```python
from build123d import *

# Parameters (mm, degrees)
SKETCH1_W           = 5.54
SKETCH1_H           = 6.3
BOSS_EXTRUDE1_DEPTH = 8.8
SKETCH2_W           = 0.8
SKETCH2_H           = 0.5
BOSS_EXTRUDE2_DEPTH = 3.2
CUT_EXTRUDE1_REACH  = 7.54
SKETCH4_W           = 2
SKETCH4_H           = 4
CUT_EXTRUDE2_DEPTH  = 3.15
CUT_EXTRUDE2_TAPER  = 10


with BuildPart() as part:
    # Sketch1 → Boss-Extrude1 (new body)
    with BuildSketch(Plane(origin=(0, 0, 0), x_dir=(1, 0, 0), z_dir=(0, 1, 0))):
        Rectangle(SKETCH1_W, SKETCH1_H)
    extrude(amount=BOSS_EXTRUDE1_DEPTH)

    # Sketch2 → Boss-Extrude2 (add)
    with BuildSketch(Plane(origin=(0, 0, 0), x_dir=(1, 0, 0), z_dir=(0, 1, 0))):
        with Locations((1.27, 0.2)):
            Rectangle(SKETCH2_W, SKETCH2_H)
        with Locations((-1.27, 0.2)):
            Rectangle(SKETCH2_W, SKETCH2_H)
    extrude(amount=-BOSS_EXTRUDE2_DEPTH)

    # Sketch3 → Cut-Extrude1 (cut, up to next)
    with BuildSketch(Plane(origin=(2.77, 0, 0), x_dir=(0, 0, -1), z_dir=(1, 0, 0)), mode=Mode.PRIVATE) as cut_extrude1_sk1:
        with BuildLine():
            ThreePointArc((-3.15, 4.7), (-2.974264069, 5.124264069), (-2.55, 5.3))
            Line((-2.55, 5.3), (-2.337822174, 5.3))
            Line((-2.337822174, 5.3), (-1.4, 8.8))
            Line((-1.4, 8.8), (-3.15, 8.8))
            Line((-3.15, 8.8), (-3.15, 4.7))
        make_face()
    cut_extrude1_tool1 = extrude(cut_extrude1_sk1.sketch, amount=-CUT_EXTRUDE1_REACH, mode=Mode.PRIVATE) & part.part
    add(cut_extrude1_tool1.solids().sort_by_distance((2.77, 7.227986, 2.489914))[0], mode=Mode.SUBTRACT)
    # Sketch3 → Cut-Extrude1 (cut, up to next)
    with BuildSketch(Plane(origin=(2.77, 0, 0), x_dir=(0, 0, -1), z_dir=(1, 0, 0)), mode=Mode.PRIVATE) as cut_extrude1_sk2:
        Polygon((3.15, 8.8), (1.4, 8.8), (3.15, 2.268911087), align=None)
    cut_extrude1_tool2 = extrude(cut_extrude1_sk2.sketch, amount=-CUT_EXTRUDE1_REACH, mode=Mode.PRIVATE) & part.part
    add(cut_extrude1_tool2.solids().sort_by_distance((2.77, 6.62297, -2.566667))[0], mode=Mode.SUBTRACT)

    # Sketch4 → Cut-Extrude2 (cut)
    with BuildSketch(Plane.XY.offset(3.15)):
        with Locations((-1.27, 2.268911087)):
            Rectangle(SKETCH4_W, SKETCH4_H)
        with Locations((1.27, 2.268911087)):
            Rectangle(SKETCH4_W, SKETCH4_H)
    extrude(amount=-CUT_EXTRUDE2_DEPTH, taper=CUT_EXTRUDE2_TAPER, mode=Mode.SUBTRACT)


solid = part.part
```
The listing builds one solid part. Answer for the finished solid, in the listing's coordinates (mm). A direction names the side the tool comes from. Coordinates: 2 decimals unless noted, no trailing zeros. Write each loop counter-clockwise with the first axis right and the second up, starting at its lowest first coordinate (ties: lowest second). Pieces come first, ordered by that corner, then holes. Notation, with made-up numbers: (0.5, 21) - (55.5, 21) arc R28 ccw to (55.5, 59) - close; hole circle Ø6 at (-9.75, -14). An arc over 180 degrees is marked (long way). One line per item, written item: value.
1) Find section A-A (y = -0.25). Give the vertices of the cut face in (x, z), and give its area (3 significant figures).
Geometry check:
outline: (-1.67, -0.45) - (-0.87, -0.45) - (-0.87, 0.05) - (-1.67, 0.05) - close; (0.87, -0.45) - (1.67, -0.45) - (1.67, 0.05) - (0.87, 0.05) - close
area: 0.800 mm2
2) Find section B-B (z = -0.25). Give the vertices of the cut face in (x, y), and give its area (3 significant figures).
Geometry check:
outline: (-2.77, 0) - (-1.67, 0) - (-1.67, -3.2) - (-0.87, -3.2) - (-0.87, 0) - (0.87, 0) - (0.87, -3.2) - (1.67, -3.2) - (1.67, 0) - (2.77, 0) - (2.77, 8.8) - (-2.77, 8.8) - close
area: 53.9 mm2
3) Find section D-D (z = 1). Count the separate pieces of the cut face and the enclosed holes in it, and give its area (3 significant figures).
Geometry check:
separate pieces: 1
enclosed holes: 2
area: 40.7 mm2
4) Consider line 1 along X through (y, z) = (-1.5, 0); line 2 along X through (y, z) = (1, 1); line 3 along Z through (x, y) = (-1.1, -0.5). Determine where each line is inside the solid, lowest interval first. Write a range as from..to.
Geometry check:
line 1: x = -1.67..-0.87, 0.87..1.67
line 2: x = -2.77..-1.89, -0.65..0.65, 1.89..2.77
line 3: z = -0.45..0.05
5) Find section C-C (x = -0.1). Give the vertices of the cut face in (y, z), and give its area (3 significant figures).
Geometry check:
outline: (0, -3.15) - (2.27, -3.15) - (8.8, -1.4) - (8.8, 1.4) - (5.3, 2.34) - (5.3, 2.55) arc R0.6 ccw to (4.7, 3.15) - (0, 3.15) - close
area: 45.2 mm2
6) This flat-tipped pin is pushed along its axis until it touches: pin 1 Ø0.9 at (x, y) = (1, -2.5) entering from -Z. Where does it stop, or does it pass through?
Geometry check:
pin 1: stops at z = -0.45
7) For a pull along X with two mould halves and no side action, classify faces 1 (the flat face through (1, 2, 0)), 2 (the flat face through (2.77, 3, 0)), 3 (the flat face through (0, 1, -3.15)) as pulls with the +X half, pulls with the -X half, needs draft (parallel to the pull), parting line crosses it, or undercut.
Geometry check:
face 1: undercut
face 2: pulls with the +X half
face 3: needs draft
8) A tool of negligible diameter and unlimited length cuts with its end or side. For faces 4 (the flat face through (-1, 2, 0)), 5 (the flat face through (0, 8.8, 0)), from which of +Z, -Z, +X, -X, +Y, -Y can it reach the whole face along a straight path? Write none if from no direction.
Geometry check:
face 4: +Z
face 5: +Z, -Z, +X, -X, +Y
